from build123d import *

# Parameters (mm, degrees)
F0_R     = 11.45
F0_R_2   = 3.826519
F0_R_3   = 2.794
F0_R_4   = 2.032
F1_DEPTH = 7


with BuildPart() as f1:
    # F0 (on Top) → F1 (new body)
    with BuildSketch(Plane.XY):
        with BuildLine():
            ThreePointArc((11.648042, -6.725), (12.991702, -3.481116), (13.45, 0))
            ThreePointArc((13.45, 0), (11.648042, 6.725), (6.725, 11.648042))
            ThreePointArc((6.725, 11.648042), (3.481116, 12.991702), (0, 13.45))
            ThreePointArc((0, 13.45), (-9.510586, 9.510586), (-13.45, 0))
            ThreePointArc((-13.45, 0), (-12.991702, -3.481116), (-11.648042, -6.725))
            ThreePointArc((-11.648042, -6.725), (-3.481116, -12.991702), (6.725, -11.648042))
            ThreePointArc((6.725, -11.648042), (9.510586, -9.510586), (11.648042, -6.725))
        make_face()
        Circle(F0_R, mode=Mode.SUBTRACT)
        with BuildLine():
            ThreePointArc((6.725, 11.648042), (11.648042, 6.725), (13.45, 0))
            ThreePointArc((13.45, 0), (12.991702, -3.481116), (11.648042, -6.725))
            Line((11.648042, -6.725), (44.823277, 12.010361))
            Line((44.823277, 12.010361), (6.725, 11.648042))
        make_face()
        with Locations((18.028694, 4.64322)):
            Circle(F0_R_2, mode=Mode.SUBTRACT)
        with Locations((26.411475, 7.009044)):
            Circle(F0_R_3, mode=Mode.SUBTRACT)
        with Locations((32.576921, 8.769555)):
            Circle(F0_R_4, mode=Mode.SUBTRACT)
        with BuildLine():
            ThreePointArc((-13.45, 0), (-9.510586, 9.510586), (0, 13.45))
            Line((0, 13.45), (-32.812916, 32.812916))
            Line((-32.812916, 32.812916), (-13.45, 0))
        make_face()
        with Locations((-13.035493, 13.291697)):
            Circle(F0_R_2, mode=Mode.SUBTRACT)
        with Locations((-19.275748, 19.368486)):
            Circle(F0_R_3, mode=Mode.SUBTRACT)
        with Locations((-23.883118, 23.827664)):
            Circle(F0_R_4, mode=Mode.SUBTRACT)
        with BuildLine():
            Line((-12.010361, -44.823277), (6.725, -11.648042))
            ThreePointArc((6.725, -11.648042), (-3.481116, -12.991702), (-11.648042, -6.725))
            Line((-11.648042, -6.725), (-12.010361, -44.823277))
        make_face()
        with Locations((-8.693803, -32.597219)):
            Circle(F0_R_4, mode=Mode.SUBTRACT)
        with Locations((-7.135727, -26.37753)):
            Circle(F0_R_3, mode=Mode.SUBTRACT)
        with Locations((-4.993201, -17.934917)):
            Circle(F0_R_2, mode=Mode.SUBTRACT)
    extrude(amount=F1_DEPTH)


solid = f1.part
Model file for the job. Use its own axes, mm. Coordinates: 2 decimals unless noted, no trailing zeros. Loops run counter-clockwise (first coordinate to the right, second up) from the corner with the lowest first, then second, coordinate; pieces in that order, holes last. Notation, with made-up numbers: (43.25, 18.25) -> (86.25, 18.25) arc R26 cw to (86.25, 52.25) -> close; hole circle Ø11 at (71, 55). An arc over 180 degrees is marked (long way). Use one line per item in the form item = value. Start each with the question number.
(1) Cut at D-D on y = 27. Give the cut face in (x, z), and give its area (3 significant figures).
(2) Probe probe 1 along Y at (x, z) = (-4, 5.25); probe 2 along X at (y, z) = (-16.5, 3.5); probe 3 along Y at (x, z) = (-19, 3). List the from-to ranges inside material, lowest first. Write a range as from..to.
(3) Cut at C-C on x = 1.5. Give the cut face in (y, z), and give its area (3 significant figures).
(4) Pull direction X, two halves, no side cores. Call faces 1 (the flat face through (-2.774, -28.468, 3.451)), 2 (the cylindrical face through (-5.49, -14.14, 3.45)), 3 (the flat face through (12, 0, 7)), 4 (the cylindrical face through (-22.79, 25.54, 3.45)): pulls with the +X half, pulls with the -X half, needs draft (parallel to the pull), parting line crosses it, or undercut.
(5) Cut at A-A on z = 4.75. Give the number of separate pieces and of enclosed holes in the cut face, and give its area (3 significant figures).
(6) Cut at B-B on y = -15. Give the cut face in (x, z).
Values:
q1.outline = (-29.38, 0) -> (-22.96, 0) -> (-22.96, 7) -> (-29.38, 7) -> close
q1.area = 44.9 mm2
q2.probe_1 = -30.64..-21.63, -14.24..-10.73, 10.73..15.81
q2.probe_2 = -11.74..-8.54, -1.45..3.98
q2.probe_3 = 9.41..16.59, 22.15..24.66
q3.outline = (-20.9, 0) -> (-11.35, 0) -> (-11.35, 7) -> (-20.9, 7) -> close; (11.35, 0) -> (13.37, 0) -> (13.37, 7) -> (11.35, 7) -> close
q3.area = 80.9 mm2
q4.face_1 = pulls with the +X half
q4.face_2 = undercut
q4.face_3 = needs draft
q4.face_4 = undercut
q5.separate_pieces = 1
q5.enclosed_holes = 10
q5.area = 804 mm2
q6.outline = (-11.73, 0) -> (-7.45, 0) -> (-7.45, 7) -> (-11.73, 7) -> close; (-2.54, 0) -> (4.83, 0) -> (4.83, 7) -> (-2.54, 7) -> close
